Could you check a few things on this drawing? It's one solid part, dimensions in mm from its lowest x, y, z. Round coordinates to 2 decimals unless told otherwise and drop trailing zeros. Write each loop counter-clockwise with the first axis right and the second up, starting at its lowest first coordinate (ties: lowest second). Pieces come first, ordered by that corner, then holes. Notation, with made-up numbers: (36.5, 15.5) -> (69.5, 15.5) arc R16 ccw to (69.5, 35.5) -> close; hole circle Ø1 at (55, 68). An arc over 180 degrees is marked (long way). Answer in a Markdown table with one row per item.
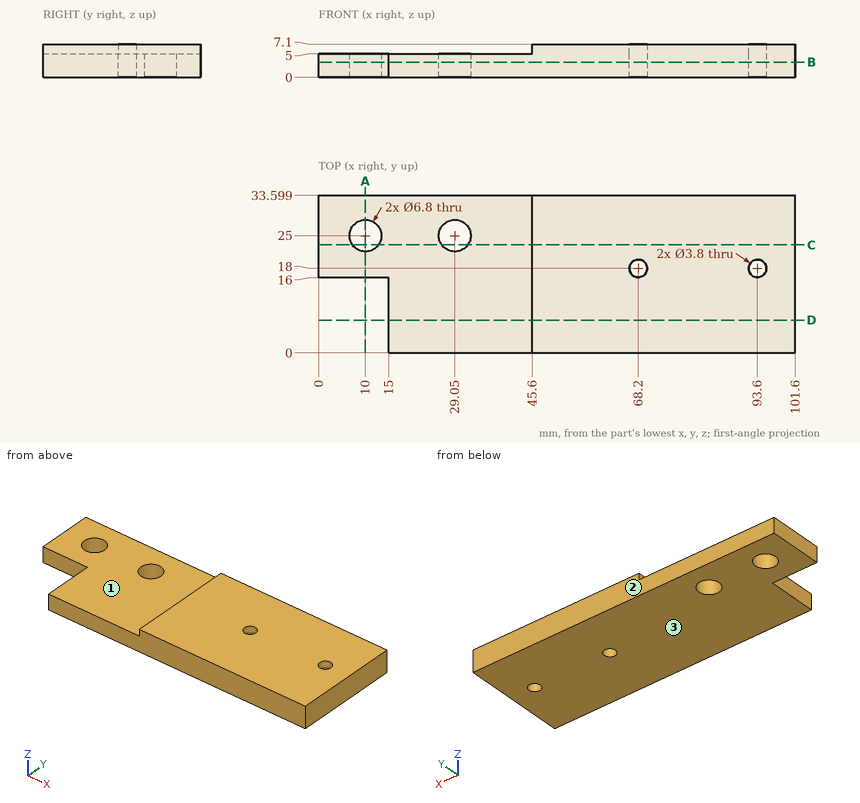
1) I want a section at C-C, the plane y = 23. List the corners of the cut face in (x, z) for me, and give its area (3 significant figures).
Response:
| item | result |
|---|---|
| outline | (0, 0) -> (7.25, 0) -> (7.25, 5) -> (0, 5) -> close; (12.75, 0) -> (26.3, 0) -> (26.3, 5) -> (12.75, 5) -> close; (31.8, 0) -> (101.6, 0) -> (101.6, 7.1) -> (45.6, 7.1) -> (45.6, 5) -> (31.8, 5) -> close |
| area | 571 mm^2 |
2) I want a section at D-D, the plane y = 7. List the corners of the cut face in (x, z) for me, and give its area (3 significant figures).
Response:
| item | result |
|---|---|
| outline | (15, 0) -> (101.6, 0) -> (101.6, 7.1) -> (45.6, 7.1) -> (45.6, 5) -> (15, 5) -> close |
| area | 551 mm^2 |
3) I need wall thicknesses on line 1 (X direction, y = 18, z = 5.85); line 2 (Y direction, x = 93.6, z = 6.05); line 3 (Y direction, x = 10, z = 1.95). Which ranges of each line are inside material? Lowest first, please. Write a range as [from, to].
Response:
| item | result |
|---|---|
| line 1 | x = [45.6, 66.3], [70.1, 91.7], [95.5, 101.6] |
| line 2 | y = [0, 16.1], [19.9, 33.6] |
| line 3 | y = [16, 21.6], [28.4, 33.6] |
4) For pin 1 (10 mm diameter, centred on x = 20.5, y = 25, fed in from +Z); pin 2 (1 mm diameter, centred on x = 75, y = 4, fed in from -Z); pin 3 (4 mm diameter, centred on y = 5, z = 1.5, fed in from -X); pin 4 (2.5 mm diameter, centred on y = 9.5, z = 6.5, fed in from -X), each with a flat end and sliding along its axis, tell me the tip position at first contact or that it passes through.
Response:
| item | result |
|---|---|
| pin 1 | stops at z = 5 |
| pin 2 | stops at z = 0 |
| pin 3 | stops at x = 15 |
| pin 4 | stops at x = 45.6 |
5) I want a section at B-B, the plane z = 3.25. List the corners of the cut face in (x, y) for me, and give its area (3 significant figures).
Response:
| item | result |
|---|---|
| outline | (0, 16) -> (15, 16) -> (15, 0) -> (101.6, 0) -> (101.6, 33.6) -> (0, 33.6) -> close; hole circle Ø6.8 at (10, 25); hole circle Ø6.8 at (29.05, 25); hole circle Ø3.8 at (68.2, 18); hole circle Ø3.8 at (93.6, 18) |
| area | 3,080 mm^2 |
6) We'd pull the mould along Z, two halves only. Please class the marked faces 1, 2 and 3: +Z half, -Z half, draft (parallel to the pull), parting line (faces both ways), or undercut.
Response:
| item | result |
|---|---|
| face 1 | +Z half |
| face 2 | draft |
| face 3 | -Z half |
7) I want a section at A-A, the plane x = 10. List the corners of the cut face in (y, z) for me.
Response:
| item | result |
|---|---|
| outline | (16, 0) -> (21.6, 0) -> (21.6, 5) -> (16, 5) -> close; (28.4, 0) -> (33.6, 0) -> (33.6, 5) -> (28.4, 5) -> close |
